The model under review builds one solid part; all positions refer to its coordinate system, in mm. Face numbers are marked on the shaded views. Coordinates: 2 decimals unless noted, no trailing zeros. Order: outer loops, then holes, each group sorted by start corner. A loop starts at its lowest first (then second) coordinate and runs counter-clockwise, first axis right, second up.
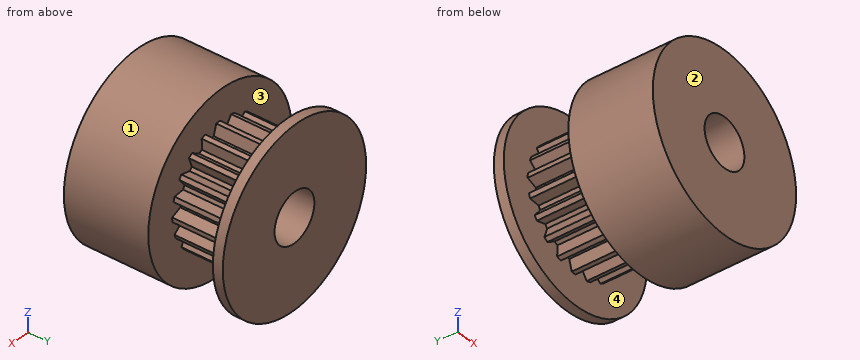
```python
from build123d import *

# Parameters (mm, degrees)
SKETCH_1_R          = 9
EXTRUDE_1_DEPTH     = 8.5
SKETCH_2_R          = 6
EXTRUDE_2_DEPTH     = 6.5
SKETCH_3_R          = 9
EXTRUDE_3_DEPTH     = 1
SKETCH_4_R          = 2.5
CUT_EXTRUDE_1_DEPTH = 17
CUT_EXTRUDE_2_DEPTH = 6.5


with BuildPart() as part:
    # 草图1 → 凸台-拉伸1 (new body)
    with BuildSketch(Plane(origin=(0, 0, 0), x_dir=(1, 0, 0), z_dir=(0, 1, 0))):
        Circle(SKETCH_1_R)
    extrude(amount=EXTRUDE_1_DEPTH)

    # 草图2 → 凸台-拉伸2 (add)
    with BuildSketch(Plane(origin=(0, 8.5, 0), x_dir=(1, 0, 0), z_dir=(0, 1, 0))):
        Circle(SKETCH_2_R)
    extrude(amount=EXTRUDE_2_DEPTH)

    # 草图3 → 凸台-拉伸3 (add)
    with BuildSketch(Plane(origin=(0, 15, 0), x_dir=(1, 0, 0), z_dir=(0, 1, 0))):
        Circle(SKETCH_3_R)
    extrude(amount=EXTRUDE_3_DEPTH)

    # 草图4 → 切除-拉伸1 (cut, through all)
    with BuildSketch(Plane(origin=(0, 16, 0), x_dir=(1, 0, 0), z_dir=(0, 1, 0))):
        Circle(SKETCH_4_R)
    extrude(amount=-CUT_EXTRUDE_1_DEPTH, mode=Mode.SUBTRACT)

    # 草图5 → 切除-拉伸2 (cut)
    with BuildSketch(Plane(origin=(0, 8.5, 0), x_dir=(1, 0, 0), z_dir=(0, 1, 0))):
        with BuildLine():
            Line((-6, 0), (-4.984088538, 0.398574263))
            ThreePointArc((-4.984088538, 0.398574263), (-4.96506054, 0.590062568), (-4.938678327, 0.780676876))
            Line((-4.938678327, 0.780676876), (-5.83314158, 1.40515455))
            ThreePointArc((-5.83314158, 1.40515455), (-5.958139369, 0.707513435), (-6, 0))
        make_face()
        with BuildLine():
            Line((-5.981863946, -0.466158487), (-4.938204626, -0.783667703))
            ThreePointArc((-4.938204626, -0.783667703), (-4.904392542, -0.973105234), (-4.863316103, -1.161101409))
            Line((-4.863316103, -1.161101409), (-5.706339098, -1.854101966))
            ThreePointArc((-5.706339098, -1.854101966), (-5.885160947, -1.168281057), (-5.981863946, -0.466158487))
        make_face()
        with BuildLine():
            Line((-5.706339098, 1.854101966), (-4.616983661, 1.91923471))
            ThreePointArc((-4.616983661, 1.91923471), (-4.539713819, 2.095470935), (-4.455719783, 2.268603363))
            Line((-4.455719783, 2.268603363), (-5.113430674, 3.13892127))
            ThreePointArc((-5.113430674, 3.13892127), (-5.447893597, 2.514051583), (-5.706339098, 1.854101966))
        make_face()
        with BuildLine():
            Line((-4.854101966, 3.526711514), (-3.797936255, 3.252027091))
            ThreePointArc((-3.797936255, 3.252027091), (-3.669988279, 3.395760008), (-3.536604341, 3.534463146))
            Line((-3.536604341, 3.534463146), (-3.893181547, 4.565428506))
            ThreePointArc((-3.893181547, 4.565428506), (-4.404370041, 4.074496845), (-4.854101966, 3.526711514))
        make_face()
        with BuildLine():
            Line((-3.526711514, 4.854101966), (-2.607120386, 4.266488403))
            ThreePointArc((-2.607120386, 4.266488403), (-2.441018717, 4.36364843), (-2.271301426, 4.454345051))
            Line((-2.271301426, 4.454345051), (-2.291840684, 5.545039791))
            ThreePointArc((-2.291840684, 5.545039791), (-2.929716059, 5.236101967), (-3.526711514, 4.854101966))
        make_face()
        with BuildLine():
            Line((-1.854101966, 5.706339098), (-1.161101409, 4.863316103))
            ThreePointArc((-1.161101409, 4.863316103), (-0.973105234, 4.904392542), (-0.783667703, 4.938204626))
            Line((-0.783667703, 4.938204626), (-0.466158487, 5.981863946))
            ThreePointArc((-0.466158487, 5.981863946), (-1.168281057, 5.885160947), (-1.854101966, 5.706339098))
        make_face()
        with BuildLine():
            Line((0, 6), (0.398574263, 4.984088538))
            ThreePointArc((0.398574263, 4.984088538), (0.590062568, 4.96506054), (0.780676876, 4.938678327))
            Line((0.780676876, 4.938678327), (1.40515455, 5.83314158))
            ThreePointArc((1.40515455, 5.83314158), (0.707513435, 5.958139369), (0, 6))
        make_face()
        with BuildLine():
            Line((1.854101966, 5.706339098), (1.91923471, 4.616983661))
            ThreePointArc((1.91923471, 4.616983661), (2.095470935, 4.539713819), (2.268603363, 4.455719783))
            Line((2.268603363, 4.455719783), (3.13892127, 5.113430674))
            ThreePointArc((3.13892127, 5.113430674), (2.514051583, 5.447893597), (1.854101966, 5.706339098))
        make_face()
        with BuildLine():
            Line((3.526711514, 4.854101966), (3.252027091, 3.797936255))
            ThreePointArc((3.252027091, 3.797936255), (3.395760008, 3.669988279), (3.534463146, 3.536604341))
            Line((3.534463146, 3.536604341), (4.565428506, 3.893181547))
            ThreePointArc((4.565428506, 3.893181547), (4.074496845, 4.404370041), (3.526711514, 4.854101966))
        make_face()
        with BuildLine():
            Line((4.854101966, 3.526711514), (4.266488403, 2.607120386))
            ThreePointArc((4.266488403, 2.607120386), (4.36364843, 2.441018717), (4.454345051, 2.271301426))
            Line((4.454345051, 2.271301426), (5.545039791, 2.291840684))
            ThreePointArc((5.545039791, 2.291840684), (5.236101967, 2.929716059), (4.854101966, 3.526711514))
        make_face()
        with BuildLine():
            Line((5.706339098, 1.854101966), (4.863316103, 1.161101409))
            ThreePointArc((4.863316103, 1.161101409), (4.904392542, 0.973105234), (4.938204626, 0.783667703))
            Line((4.938204626, 0.783667703), (5.981863946, 0.466158487))
            ThreePointArc((5.981863946, 0.466158487), (5.885160947, 1.168281057), (5.706339098, 1.854101966))
        make_face()
        with BuildLine():
            Line((6, 0), (4.984088538, -0.398574263))
            ThreePointArc((4.984088538, -0.398574263), (4.96506054, -0.590062568), (4.938678327, -0.780676876))
            Line((4.938678327, -0.780676876), (5.83314158, -1.40515455))
            ThreePointArc((5.83314158, -1.40515455), (5.958139369, -0.707513435), (6, 0))
        make_face()
        with BuildLine():
            Line((5.706339098, -1.854101966), (4.616983661, -1.91923471))
            ThreePointArc((4.616983661, -1.91923471), (4.539713819, -2.095470935), (4.455719783, -2.268603363))
            Line((4.455719783, -2.268603363), (5.113430674, -3.13892127))
            ThreePointArc((5.113430674, -3.13892127), (5.447893597, -2.514051583), (5.706339098, -1.854101966))
        make_face()
        with BuildLine():
            Line((4.854101966, -3.526711514), (3.797936255, -3.252027091))
            ThreePointArc((3.797936255, -3.252027091), (3.669988279, -3.395760008), (3.536604341, -3.534463146))
            Line((3.536604341, -3.534463146), (3.893181547, -4.565428506))
            ThreePointArc((3.893181547, -4.565428506), (4.404370041, -4.074496845), (4.854101966, -3.526711514))
        make_face()
        with BuildLine():
            Line((3.526711514, -4.854101966), (2.607120386, -4.266488403))
            ThreePointArc((2.607120386, -4.266488403), (2.441018717, -4.36364843), (2.271301426, -4.454345051))
            Line((2.271301426, -4.454345051), (2.291840684, -5.545039791))
            ThreePointArc((2.291840684, -5.545039791), (2.929716059, -5.236101967), (3.526711514, -4.854101966))
        make_face()
        with BuildLine():
            Line((1.854101966, -5.706339098), (1.161101409, -4.863316103))
            ThreePointArc((1.161101409, -4.863316103), (0.973105234, -4.904392542), (0.783667703, -4.938204626))
            Line((0.783667703, -4.938204626), (0.466158487, -5.981863946))
            ThreePointArc((0.466158487, -5.981863946), (1.168281057, -5.885160947), (1.854101966, -5.706339098))
        make_face()
        with BuildLine():
            Line((0, -6), (-0.398574263, -4.984088538))
            ThreePointArc((-0.398574263, -4.984088538), (-0.590062568, -4.96506054), (-0.780676876, -4.938678327))
            Line((-0.780676876, -4.938678327), (-1.40515455, -5.83314158))
            ThreePointArc((-1.40515455, -5.83314158), (-0.707513435, -5.958139369), (0, -6))
        make_face()
        with BuildLine():
            Line((-1.854101966, -5.706339098), (-1.91923471, -4.616983661))
            ThreePointArc((-1.91923471, -4.616983661), (-2.095470935, -4.539713819), (-2.268603363, -4.455719783))
            Line((-2.268603363, -4.455719783), (-3.13892127, -5.113430674))
            ThreePointArc((-3.13892127, -5.113430674), (-2.514051583, -5.447893597), (-1.854101966, -5.706339098))
        make_face()
        with BuildLine():
            Line((-3.526711514, -4.854101966), (-3.252027091, -3.797936255))
            ThreePointArc((-3.252027091, -3.797936255), (-3.395760008, -3.669988279), (-3.534463146, -3.536604341))
            Line((-3.534463146, -3.536604341), (-4.565428506, -3.893181547))
            ThreePointArc((-4.565428506, -3.893181547), (-4.074496845, -4.404370041), (-3.526711514, -4.854101966))
        make_face()
        with BuildLine():
            Line((-4.854101966, -3.526711514), (-4.266488403, -2.607120386))
            ThreePointArc((-4.266488403, -2.607120386), (-4.36364843, -2.441018717), (-4.454345051, -2.271301426))
            Line((-4.454345051, -2.271301426), (-5.545039791, -2.291840684))
            ThreePointArc((-5.545039791, -2.291840684), (-5.236101967, -2.929716059), (-4.854101966, -3.526711514))
        make_face()
    extrude(amount=CUT_EXTRUDE_2_DEPTH, mode=Mode.SUBTRACT)


solid = part.part
```
(1) We need section A-A, the plane y = 2.5. Write out the cut boundary in (x, z).
A:
outline: circle Ø18 at (0, 0); hole circle Ø5 at (0, 0)
(2) Wall thickness on probe 1 along Y at (x, z) = (7.25, -1); probe 2 along X at (y, z) = (4, 0); probe 3 along Z at (x, y) = (-4.75, 9): over which ranges is each line inside the solid? List them lowest first.
A:
probe 1: y = 0 to 8.5, 15 to 16
probe 2: x = -9 to -2.5, 2.5 to 9
probe 3: z = -3.5 to -2.66, -1.91 to 2.28, 3.36 to 3.67
(3) Draft analysis for pull direction Y (two halves, no side actions). For the marked faces 1, 2, 3 and 4, state which applies: released by +Y, released by -Y, zero draft, split by the parting line, or undercut.
A:
face 1: zero draft
face 2: released by -Y
face 3: undercut
face 4: undercut
(4) For pin 1 Ø1.5 at (y, z) = (5, -0.5) entering from -X; pin 2 Ø3 at (y, z) = (2, 4.5) entering from +X; pin 3 Ø1 at (y, z) = (12, 3.5) entering from +X, all flat-tipped, find the tip position at first contact; note any pin that passes through.
A:
pin 1: stops at x = -9
pin 2: stops at x = 8.49
pin 3: stops at x = 5.11
